Design review of the part shown in the three views and the two pictorial views. Dimensions are in mm from the part's minimum x, y and z. A direction names the side the tool comes from. Round coordinates to 2 decimals unless told otherwise and drop trailing zeros. Order: outer loops, then holes, each group sorted by start corner. A loop starts at its lowest first (then second) coordinate and runs counter-clockwise, first axis right, second up. Notation, with made-up numbers: (41, -24) - (65, -24) arc R12 cw to (65, -1) - close; hole circle Ø8 at (19.25, 77). An arc over 180 degrees is marked (long way). Use CSV: the item, a comma, the result in double quotes.
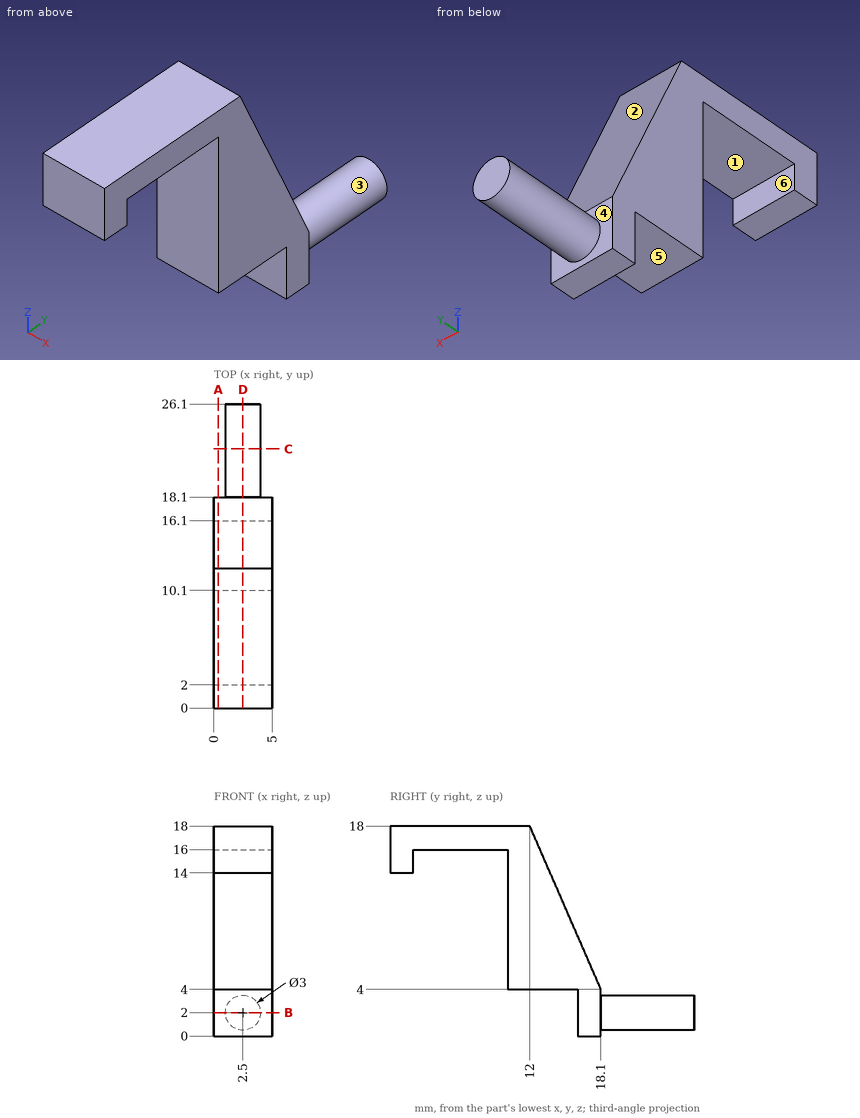
1) We need section A-A (x = 0.4). Give the boundary of the cut face in (y, z).
Data:
outline,"(0, 14) - (2, 14) - (2, 16) - (10.1, 16) - (10.1, 4) - (16.1, 4) - (16.1, 0) - (18.1, 0) - (18.1, 4) - (12, 18) - (0, 18) - close"
2) We need section B-B (z = 2). Give the boundary of the cut face in (x, y).
Data:
outline,"(0, 16.1) - (5, 16.1) - (5, 18.1) - (4, 18.1) - (4, 26.1) - (1, 26.1) - (1, 18.1) - (0, 18.1) - close"
3) For the marked faces 4, 5 and 6, list the 3-axis set-ups (+Z, -Z, +X, -X, +Y, -Y) from which the entire face can be reached by the end or side of a thin tool; tool diameter is ignored.
Data:
face 4,"+Y"
face 5,"-Z, +X, -X, -Y"
face 6,"-Z, +X, -X"
4) We need section D-D (x = 2.5). Give the boundary of the cut face in (y, z).
Data:
outline,"(0, 14) - (2, 14) - (2, 16) - (10.1, 16) - (10.1, 4) - (16.1, 4) - (16.1, 0) - (18.1, 0) - (18.1, 0.5) - (26.1, 0.5) - (26.1, 3.5) - (18.1, 3.5) - (18.1, 4) - (12, 18) - (0, 18) - close"
5) We need section C-C (y = 22.25). Give the boundary of the cut face in (x, z).
Data:
outline,"circle Ø3 at (2.5, 2)"
6) The part is to be moulded in two halves that separate along Y. For the marked faces 1, 2 and 3, say which applies: +Y half, -Y half, draft (parallel to the pull), parting line (faces both ways), or undercut.
Data:
face 1,"undercut"
face 2,"+Y half"
face 3,"draft"
7) To check wall thickness, follow L1, parallel to Y at x = 2.75, z = 1; L2, parallel to Y at x = 3.5, z = 3.5; L3, parallel to Z at x = 3.6, y = 2.25. State the ranges of each line that lie inside material, in increasing order. Write a range as from..to.
Data:
L1,"y = 16.1..26.1"
L2,"y = 16.1..18.1"
L3,"z = 16..18"
8) Insertion check: pin 1 Ø2.5 at (x, z) = (2, 8.5) entering from -Y; pin 2 Ø1.5 at (x, y) = (2.5, 15) entering from +Z; pin 3 Ø0.6 at (x, y) = (1.5, 0.5) entering from -Z; pin 4 Ø5 at (y, z) = (8.5, 11.5) entering from -X. Each pin has a flat end and moves straight along its axis. Give the tip position at first contact, or say it passes through.
Data:
pin 1,"stops at y = 10.1"
pin 2,"stops at z = 12.84"
pin 3,"stops at z = 14"
pin 4,"stops at x = 0"
